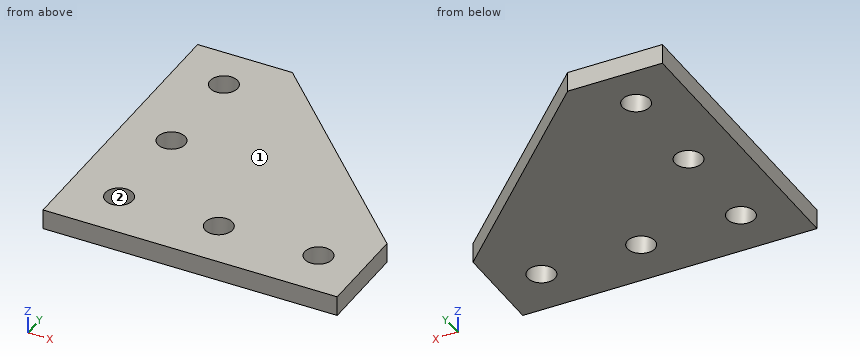
```python
from build123d import *

# Parameters (mm, degrees)
SKETCH1_R           = 2.75
BOSS_EXTRUDE1_DEPTH = 2


with BuildPart() as part:
    # Sketch1 → Boss-Extrude1 (new body, symmetric)
    with BuildSketch(Plane.XY):
        Polygon((0, 0), (0, 59), (19, 59), (59, 19), (59, 0), align=None)
        with Locations((10, 10)):
            Circle(SKETCH1_R, mode=Mode.SUBTRACT)
        with Locations((10, 30)):
            Circle(SKETCH1_R, mode=Mode.SUBTRACT)
        with Locations((10, 50)):
            Circle(SKETCH1_R, mode=Mode.SUBTRACT)
        with Locations((30, 10)):
            Circle(SKETCH1_R, mode=Mode.SUBTRACT)
        with Locations((50, 10)):
            Circle(SKETCH1_R, mode=Mode.SUBTRACT)
    extrude(amount=BOSS_EXTRUDE1_DEPTH, both=True)


solid = part.part
```
CAD build for the part. Positions are in the model's coordinates, mm. Face numbers are marked on the shaded views. Coordinates: 2 decimals unless noted, no trailing zeros. Order: outer loops, then holes, each group sorted by start corner. A loop starts at its lowest first (then second) coordinate and runs counter-clockwise, first axis right, second up. Notation, with made-up numbers: (-20.75, 36.25) -> (8.25, 36.25) arc R23 cw to (8.25, 66.25) -> close; hole circle Ø5 at (42, 31.25). An arc over 180 degrees is marked (long way). Use one line per item in the form item = value. Start each with the question number.
1) Drop a flat-ended pin along its axis: pin 1 (2 mm diameter, centred on y = 30.5, z = 1, fed in from +X). Give the stop position or say it passes through.
2) Band-saw the part on C-C on x = 10. Give the cut face in (y, z).
3) Band-saw the part on D-D on z = -0.8. Give the cut face in (x, y).
4) Drill centre lines: L1, parallel to Y at x = 10, z = 0.65; L2, parallel to X at y = 11.5, z = -0.5; L3, parallel to Y at x = 50, z = 1.1. Where is each one in solid material? Low to high. Write a range as [from, to].
5) Band-saw the part on B-B on y = 50. Give the cut face in (x, z), then the cut area to 3 significant figures.
6) Band-saw the part on A-A on x = 30. Give the cut face in (y, z), then the cut area to 3 significant figures.
7) Pull direction X, two halves, no side cores. Call the marked faces 1 and 2: +X half, -X half, draft (parallel to the pull), parting line (faces both ways), or undercut.
Entries:
q1.pin_1 = 48.5
q2.outline = (0, -2) -> (7.25, -2) -> (7.25, 2) -> (0, 2) -> close; (12.75, -2) -> (27.25, -2) -> (27.25, 2) -> (12.75, 2) -> close; (32.75, -2) -> (47.25, -2) -> (47.25, 2) -> (32.75, 2) -> close; (52.75, -2) -> (59, -2) -> (59, 2) -> (52.75, 2) -> close
q3.outline = (0, 0) -> (59, 0) -> (59, 19) -> (19, 59) -> (0, 59) -> close; hole circle Ø5.5 at (10, 10); hole circle Ø5.5 at (10, 30); hole circle Ø5.5 at (10, 50); hole circle Ø5.5 at (30, 10); hole circle Ø5.5 at (50, 10)
q4.L1 = [0, 7.25], [12.75, 27.25], [32.75, 47.25], [52.75, 59]
q4.L2 = [0, 7.7], [12.3, 27.7], [32.3, 47.7], [52.3, 59]
q4.L3 = [0, 7.25], [12.75, 28]
q5.outline = (0, -2) -> (7.25, -2) -> (7.25, 2) -> (0, 2) -> close; (12.75, -2) -> (28, -2) -> (28, 2) -> (12.75, 2) -> close
q5.area = 90.0 mm2
q6.outline = (0, -2) -> (7.25, -2) -> (7.25, 2) -> (0, 2) -> close; (12.75, -2) -> (48, -2) -> (48, 2) -> (12.75, 2) -> close
q6.area = 170 mm2
q7.face_1 = draft
q7.face_2 = undercut
